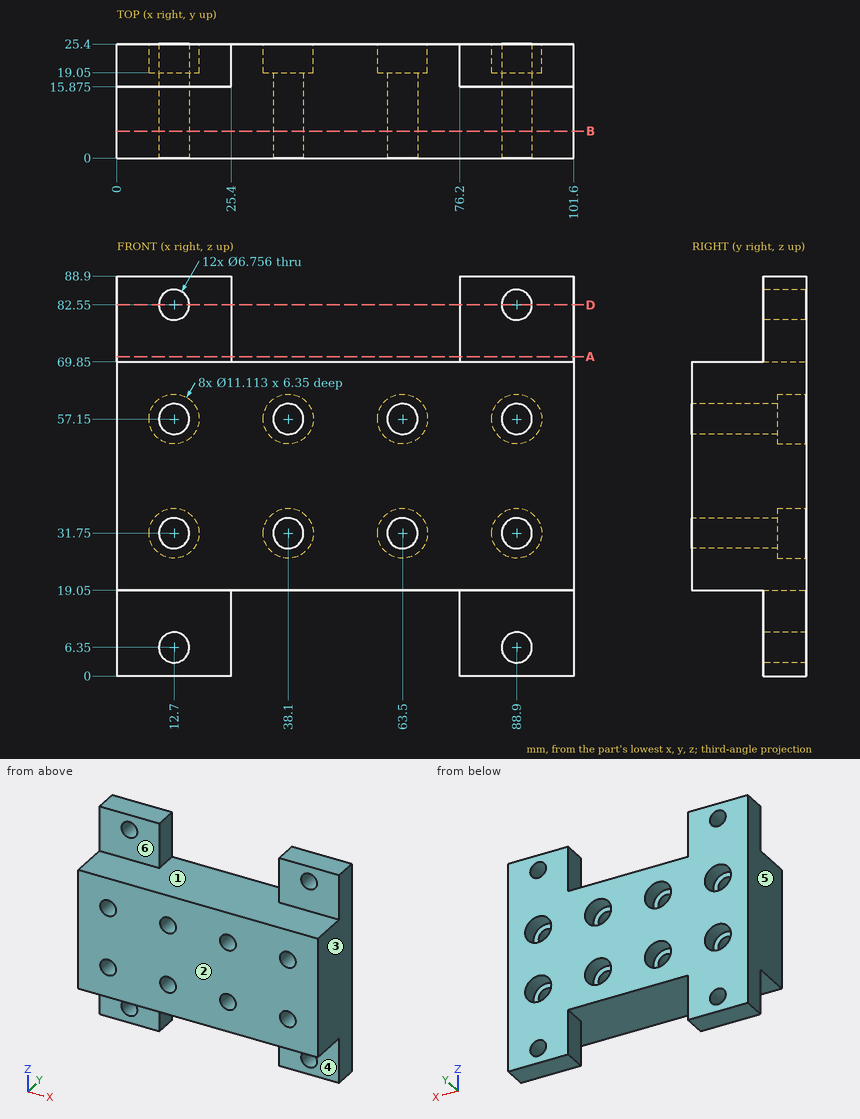
Verification items for this drawing (mm, ordinates from the low corner). A direction names the side the tool comes from. Coordinates: 2 decimals unless noted, no trailing zeros. Order: outer loops, then holes, each group sorted by start corner. A loop starts at its lowest first (then second) coordinate and runs counter-clockwise, first axis right, second up. Notation, with made-up numbers: M 21.5,71 L 32.5,71 A20 cw 32.5,86 Z; hole C -18.5,-23 d4. An arc over 180 degrees is marked long. Write each question's results on one line, items separated by ' | '.
1) Section check A-A on z = 71. Record the cut outline in (x, y) (1 decimal), plus the area to 3 significant figures.
Solved:
outline: M 0,15.9 L 25.4,15.9 L 25.4,25.4 L 0,25.4 Z; M 76.2,15.9 L 101.6,15.9 L 101.6,25.4 L 76.2,25.4 Z | area: 484 mm²
2) Gauge pin test, flat ends, axial feed: pin 1 Ø9.5 at (x, z) = (91.5, 80) entering from -Y (1 decimal); pin 2 Ø8 at (x, z) = (63.5, 31.75) entering from +Y; pin 3 Ø6 at (x, y) = (89.5, 8.5) entering from +Z; pin 4 Ø6 at (x, z) = (88.9, 6.35) entering from +Y. Record the tip position at first contact, or that the pin passes through.
Solved:
pin 1: stops at y = 15.9 | pin 2: stops at y = 19.05 | pin 3: stops at z = 69.85 | pin 4: passes through
3) Release check for a two-part mould opening along X. For the marked faces 1, 2 and 3 record: pulls with the +X half, pulls with the -X half, needs draft (parallel to the pull), parting line crosses it, or undercut.
Solved:
face 1: undercut | face 2: needs draft | face 3: pulls with the +X half
4) Section check D-D on z = 82.55. Record the cut outline in (x, y) (1 decimal).
Solved:
outline: M 0,15.9 L 9.3,15.9 L 9.3,25.4 L 0,25.4 Z; M 16.1,15.9 L 25.4,15.9 L 25.4,25.4 L 16.1,25.4 Z; M 76.2,15.9 L 85.5,15.9 L 85.5,25.4 L 76.2,25.4 Z; M 92.3,15.9 L 101.6,15.9 L 101.6,25.4 L 92.3,25.4 Z
5) Section check B-B on y = 6. Give the number of separate pieces and of enclosed holes in the cut face, plus the area to 3 significant figures.
Solved:
separate pieces: 1 | enclosed holes: 8 | area: 4,870 mm²
6) Scan lines: line 1 along Z through (x, y) = (38.1, 10.5); line 2 along Z through (x, y) = (88.9, 24.25); line 3 along Z through (x, y) = (63.5, 22.25). Record each from-to range of solid material in increasing order. Write a range as [from, to].
Solved:
line 1: z = [19.05, 28.37], [35.13, 53.77], [60.53, 69.85] | line 2: z = [0, 2.97], [9.73, 26.19], [37.31, 51.59], [62.71, 79.17], [85.93, 88.9] | line 3: z = [19.05, 26.19], [37.31, 51.59], [62.71, 69.85]
7) Access from +Z, -Z, +X, -X, +Y, -Y to the whole of each face (thin tool, end or side, straight path). Record for the marked faces 4, 5 and 6.
Solved:
face 4: -Z, +X, -X, -Y | face 5: +Z, -Z, -X, +Y, -Y | face 6: +Z, +X, -X, -Y
